CAD build for the part. Positions are in the model's coordinates, mm. Face numbers are marked on the shaded views. A direction names the side the tool comes from. Coordinates: 2 decimals unless noted, no trailing zeros. Write each loop counter-clockwise with the first axis right and the second up, starting at its lowest first coordinate (ties: lowest second). Pieces come first, ordered by that corner, then holes. Notation, with made-up numbers: M 31.25,26.25 L 85.25,26.25 A26 ccw 85.25,53.25 Z; hole C 82.5,-34.5 d2. An arc over 180 degrees is marked long. Answer as CSV lines item,"result". Start each with the question number.
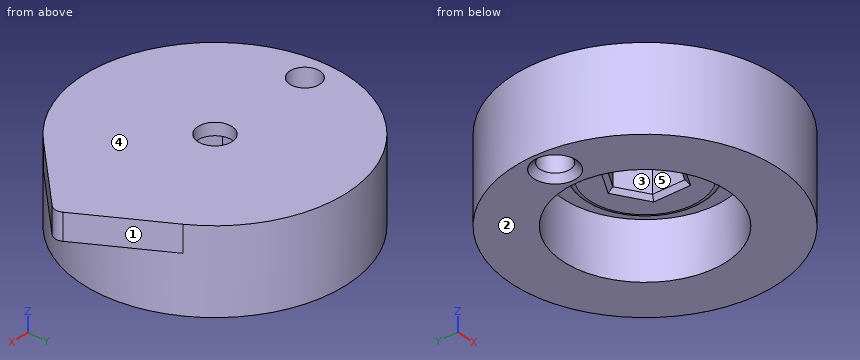
```python
from build123d import *

# Parameters (mm, degrees)
SKETCH2_R               = 32.5
BOSS_EXTRUDE1_DEPTH     = 6
SKETCH3_R               = 32.5
BOSS_EXTRUDE2_DEPTH     = 2
CHAMFER1_SIZE           = 2
CUT_EXTRUDE1_DEPTH      = 6.5
SKETCH5_R               = 4.2
CUT_EXTRUDE2_DEPTH      = 70.12488698
CUT_EXTRUDE3_DEPTH      = 70.079664157
SKETCH8_R               = 15
BOSS_EXTRUDE3_DEPTH     = 3
BOSS_EXTRUDE4_START     = 3
SKETCH9_R               = 4.2
BOSS_EXTRUDE4_DEPTH     = 3
CUT_EXTRUDE5_START      = -3
SKETCH10_R              = 32.5
CUT_EXTRUDE5_DEPTH      = 3
FILLET1_R               = 1.5
SKETCH11_R              = 32.5
BOSS_EXTRUDE5_DEPTH     = 1.5
SKETCH12_R              = 4.2
CUT_EXTRUDE6_DEPTH      = 70.282032303
CHAMFER2_SIZE           = 1
BOSS_EXTRUDE6_DEPTH     = 6.5
BOSS_EXTRUDE8_START     = -6.5
BOSS_EXTRUDE8_DEPTH     = 6.5
BOSS_EXTRUDE10_START    = 14
SKETCH16_R              = 32.5
SKETCH16_R_2            = 20
SKETCH16_R_3            = 3.7
BOSS_EXTRUDE10_DEPTH    = 14
CHAMFER3_SIZE           = 1.5
CUT_EXTRUDE7_DEPTH      = 77.342976101
CUT_EXTRUDE7_DEPTH_BACK = 77.342976101
SKETCH17_R              = 3.7


with BuildPart() as part:
    # Sketch2 → Boss-Extrude1 (new body)
    with BuildSketch(Plane.XY.offset(1)):
        with Locations((23.5, 7.5)):
            Circle(SKETCH2_R)
        with BuildLine():
            Line((-3.5, 0), (-3.5, 15))
            ThreePointArc((-3.5, 15), (0, 18.5), (3.5, 15))
            Line((3.5, 15), (3.5, 0))
            ThreePointArc((3.5, 0), (0, -3.5), (-3.5, 0))
        make_face(mode=Mode.SUBTRACT)
    extrude(amount=BOSS_EXTRUDE1_DEPTH)

    # Sketch3 → Boss-Extrude2 (add)
    with BuildSketch(Plane.XY.offset(7)):
        with Locations((23.5, 7.5)):
            Circle(SKETCH3_R)
    extrude(amount=BOSS_EXTRUDE2_DEPTH)

    # Chamfer1
    chamfer1_edges = [part.edges().sort_by_distance(p)[0] for p in [
        (-3.5, 7.5, 1),
        (0, -3.5, 1),
        (3.5, 7.5, 1),
        (0, 18.5, 1),
    ]]
    chamfer(chamfer1_edges, length=CHAMFER1_SIZE)

    # Sketch4 → Cut-Extrude1 (cut)
    with BuildSketch(Plane(origin=(0, 0, 1), x_dir=(-1, 0, 0), z_dir=(0, 0, -1))):
        Polygon((-23.5, 15.467433715), (-30.4, 11.483716857), (-30.4, 3.516283143), (-23.5, -0.467433715), (-16.6, 3.516283143), (-16.6, 11.483716857), align=None)
    extrude(amount=-CUT_EXTRUDE1_DEPTH, mode=Mode.SUBTRACT)

    # Sketch5 → Cut-Extrude2 (cut, through all)
    with BuildSketch(Plane(origin=(0, 0, 7.5), x_dir=(-1, 0, 0), z_dir=(0, 0, -1))):
        with Locations((-23.5, 7.5)):
            Circle(SKETCH5_R)
    extrude(amount=-CUT_EXTRUDE2_DEPTH, mode=Mode.SUBTRACT)

    # Sketch6 → Cut-Extrude3 (cut, through all)
    with BuildSketch(Plane(origin=(0, 0, 7), x_dir=(-1, 0, 0), z_dir=(0, 0, -1))):
        with BuildLine():
            Line((-3.5, 15), (-3.5, 0))
            ThreePointArc((-3.5, 0), (0, -3.5), (3.5, 0))
            Line((3.5, 0), (3.5, 15))
            ThreePointArc((3.5, 15), (0, 18.5), (-3.5, 15))
        make_face()
    extrude(amount=-CUT_EXTRUDE3_DEPTH, mode=Mode.SUBTRACT)

    # Sketch8 → Boss-Extrude3 (add)
    with BuildSketch(Plane(origin=(0, 0, 1), x_dir=(-1, 0, 0), z_dir=(0, 0, -1))):
        with Locations(Location((-23.5, 7.5, 0), (0, 0, 180))):
            Circle(SKETCH8_R)
        Polygon((-16.6, 3.516283143), (-16.6, 11.483716857), (-23.5, 15.467433715), (-30.4, 11.483716857), (-30.4, 3.516283143), (-23.5, -0.467433715), align=None, mode=Mode.SUBTRACT)
    extrude(amount=BOSS_EXTRUDE3_DEPTH)

    # Sketch9 → Boss-Extrude4 (add)
    with BuildSketch(Plane(origin=(0, 0, 7.5), x_dir=(-1, 0, 0), z_dir=(0, 0, -1)).offset(BOSS_EXTRUDE4_START)):
        Polygon((-16.6, 11.483716857), (-23.5, 15.467433715), (-30.4, 11.483716857), (-30.4, 3.516283143), (-23.5, -0.467433715), (-16.6, 3.516283143), align=None)
        with Locations((-23.5, 7.5)):
            Circle(SKETCH9_R, mode=Mode.SUBTRACT)
    extrude(amount=-BOSS_EXTRUDE4_DEPTH)

    # Sketch10 → Cut-Extrude5 (cut)
    with BuildSketch(Plane.XY.offset(9).offset(CUT_EXTRUDE5_START)):
        with Locations((23.5, 7.5)):
            Circle(SKETCH10_R)
    extrude(amount=CUT_EXTRUDE5_DEPTH, mode=Mode.SUBTRACT)

    # Fillet1
    fillet1_edges = [part.edges().sort_by_distance(p)[0] for p in [
        (8.5, 7.5, -2),
    ]]
    fillet(fillet1_edges, radius=FILLET1_R)

    # Sketch11 → Boss-Extrude5 (add)
    with BuildSketch(Plane.XY.offset(6)):
        with Locations((23.5, 7.5)):
            Circle(SKETCH11_R)
        with BuildLine():
            Line((3.5, 15), (3.5, 0))
            ThreePointArc((3.5, 0), (0, -3.5), (-3.5, 0))
            Line((-3.5, 0), (-3.5, 15))
            ThreePointArc((-3.5, 15), (0, 18.5), (3.5, 15))
        make_face(mode=Mode.SUBTRACT)
    extrude(amount=BOSS_EXTRUDE5_DEPTH)

    # Sketch12 → Cut-Extrude6 (cut, through all)
    with BuildSketch(Plane(origin=(0, 0, 6), x_dir=(-1, 0, 0), z_dir=(0, 0, -1))):
        with Locations((-23.5, 7.5)):
            Circle(SKETCH12_R)
    extrude(amount=-CUT_EXTRUDE6_DEPTH, mode=Mode.SUBTRACT)

    # Chamfer2
    chamfer2_edges = [part.edges().sort_by_distance(p)[0] for p in [
        (20.05, 1.524424714, -2),
        (16.6, 7.5, -2),
        (20.05, 13.475575286, -2),
        (26.95, 13.475575286, -2),
        (30.4, 7.5, -2),
        (26.95, 1.524424714, -2),
    ]]
    chamfer(chamfer2_edges, length=CHAMFER2_SIZE)

    # Sketch13 → Boss-Extrude6 (add)
    with BuildSketch(Plane(origin=(0, 0, 1), x_dir=(-1, 0, 0), z_dir=(0, 0, -1))):
        with BuildLine():
            Line((-51.749638846, 23.568848902), (-63.173049142, 3.4860653))
            ThreePointArc((-63.173049142, 3.4860653), (-63.475854367, 1.903380389), (-62.750057959, 0.464699706))
            Line((-62.750057959, 0.464699706), (-46.250753464, -15.708903826))
            ThreePointArc((-46.250753464, -15.708903826), (-55.686106767, 2.993945053), (-51.749638846, 23.568848902))
        make_face()
    extrude(amount=-BOSS_EXTRUDE6_DEPTH)

    # Sketch15 → Boss-Extrude8 (add)
    with BuildSketch(Plane.XY.offset(7.5).offset(BOSS_EXTRUDE8_START)):
        with BuildLine():
            Line((46.250753464, -15.708903826), (62.750057959, 0.464699706))
            ThreePointArc((62.750057959, 0.464699706), (63.475854367, 1.903380389), (63.173049142, 3.4860653))
            Line((63.173049142, 3.4860653), (51.749638846, 23.568848902))
            ThreePointArc((51.749638846, 23.568848902), (-8.686106767, 12.006054947), (46.250753464, -15.708903826))
        make_face()
        Polygon((23.5, -0.467433715), (16.6, 3.516283143), (16.6, 11.483716857), (23.5, 15.467433715), (30.4, 11.483716857), (30.4, 3.516283143), align=None, mode=Mode.SUBTRACT)
    extrude(amount=BOSS_EXTRUDE8_DEPTH)

    # Sketch16 → Boss-Extrude10 (add)
    with BuildSketch(Plane(origin=(0, 0, 1), x_dir=(-1, 0, 0), z_dir=(0, 0, -1)).offset(BOSS_EXTRUDE10_START)):
        with Locations((-23.5, 7.5)):
            Circle(SKETCH16_R)
        with Locations((-23.5, 7.5)):
            Circle(SKETCH16_R_2, mode=Mode.SUBTRACT)
        with Locations((2.75, 7.5)):
            Circle(SKETCH16_R_3, mode=Mode.SUBTRACT)
    extrude(amount=-BOSS_EXTRUDE10_DEPTH)

    # Chamfer3
    chamfer3_edges = [part.edges().sort_by_distance(p)[0] for p in [
        (0.95, 7.5, -13),
    ]]
    chamfer(chamfer3_edges, length=CHAMFER3_SIZE)

    # Sketch17 → Cut-Extrude7 (cut, two sides: drawn at the far end of the back side and taken through both)
    with BuildSketch(Plane(origin=(0, 0, 1), x_dir=(-1, 0, 0), z_dir=(0, 0, -1)).offset(-CUT_EXTRUDE7_DEPTH_BACK)):
        with Locations((2.75, 7.5)):
            Circle(SKETCH17_R)
    extrude(amount=CUT_EXTRUDE7_DEPTH + CUT_EXTRUDE7_DEPTH_BACK, mode=Mode.SUBTRACT)


solid = part.part
```
1) Band-saw the part on C-C, the plane z = -8. List the corners of the cut face in (x, y).
2) Pin check, flat tips, straight feed: P1, Ø10, axis at y = 1.5, z = -7, coming from the -X side; P2, Ø4.5, axis at x = -2.75, y = 7.5, coming from the -Z side; P3, Ø24, axis at x = 23.5, y = 7.5, coming from the -Z side; P4, Ø1.5, axis at x = 39, z = -5, coming from the -Y side. Stop position of each tip, or through.
3) Tool access for the marked faces 4 and 5: list every direction of +Z, -Z, +X, -X, +Y, -Y with a clear straight run to the whole face (end or side of a thin tool).
4) Two-plate mould, pull along Y, no slides. Class the marked faces 1, 2 and 3: pulls with the +Y half, pulls with the -Y half, needs draft (parallel to the pull), parting line crosses it, or undercut.
5) Band-saw the part on D-D, the plane x = 39.5. List the corners of the cut face in (y, z).
6) Band-saw the part on B-B, the plane y = 7.5. State how many separate pieces and enclosed holes the cut face has, plus the area to 3 significant figures.
7) Band-saw the part on A-A, the plane x = -2.75. List the corners of the cut face in (y, z), plus the area to 3 significant figures.
8) Probe L1, parallel to Y at x = 23.5, z = -8.5; L2, parallel to Y at x = 23.5, z = 5.85; L3, parallel to Y at x = 21, z = 0. List the from-to ranges inside material, lowest first. Write a range as [from, to].
Result sheet:
1,outline,"C 23.5,7.5 d65; hole C -2.75,7.5 d7.4; hole C 23.5,7.5 d40"
2,P1,"stops at x = -8.98"
2,P2,"passes through"
2,P3,"stops at z = -2"
2,P4,"stops at y = -21.46"
3,face 4,"+Z, +X, -X, +Y, -Y"
3,face 5,"-Z"
4,face 1,"pulls with the +Y half"
4,face 2,"needs draft"
4,face 3,"undercut"
5,outline,"M -20.79,-13 L -4.5,-13 L -4.5,1 L 19.5,1 L 19.5,-13 L 35.79,-13 L 35.79,7.5 L -20.79,7.5 Z"
6,separate pieces,"3"
6,enclosed holes,"0"
6,area,"623 mm²"
7,outline,"M -11.66,-13 L 2.3,-13 L 3.8,-11.5 L 3.8,7.5 L -11.66,7.5 Z; M 11.2,-11.5 L 12.7,-13 L 26.66,-13 L 26.66,7.5 L 11.2,7.5 Z"
7,area,"632 mm²"
8,L1,"y = [-25, -12.5], [27.5, 40]"
8,L2,"y = [-25, 3.3], [11.7, 40]"
8,L3,"y = [-24.9, -12.34], [-7.29, 0.98], [14.02, 22.29], [27.34, 39.9]"
